Autodesk Fusion 360 part; units mm, degrees
sketch "Sketch1" plane through (0, 0, 0) normal (0, 0, 1) x (1, 0, 0)
  circle A0 centre (0, 0) radius 11
  dimension "d1" = 22
extrude "Extrude1" add sketch "Sketch1" along normal blind 2.5
sketch "Sketch2" plane through (0, 0, 2.5) normal (0, 0, 1) x (-1, 0, 0)
  circle A0 centre (0, 0) radius 11
  circle A1 centre (0, 0) radius 5.5
  dimension "d4" = 11
extrude "Extrude2" add sketch "Sketch2" along normal blind 8 contours A1
sketch "Sketch3" plane through (0, 0, 2.5) normal (0, 0, 1) x (-1, 0, 0)
  circle A0 centre (0, 0) radius 5.5
  circle A1 centre (0, 0) radius 11
  circle A2 centre (5.6569, -5.6569) radius 1.4
  circle A3 centre (5.6569, 5.6569) radius 1.4
  circle A4 centre (-5.6569, 5.6569) radius 1.4
  circle A5 centre (-5.6569, -5.6569) radius 1.4
  line L0 (0, 0) -> (7.7782, -7.7782) construction
  line L1 (0, 0) -> (11, 0) construction
  dimension "d7" = 2.8
  dimension "d8" = 8
  dimension "d10" = 360
  dimension "d27" = 45
extrude "Extrude3" cut sketch "Sketch3" against normal through all contours A2 | A3 | A4 | A5
sketch "Sketch4" plane through (0, 0, 10.5) normal (0, 0, 1) x (-1, 0, 0)
  circle A0 centre (0, 0) radius 5.5
  circle A1 centre (0, 0) radius 1.1
  dimension "d12" = 2.2
extrude "Extrude4" cut sketch "Sketch4" against normal through all contours A1
chamfer "Chamfer1" distance 3 angle 45 1 edges at (5.1278, 1.9889, 10.5)
Build history of the part. All positions in model axes, mm. A direction names the side the tool comes from. Give positions to 0.01 mm unless a question says otherwise; leave off trailing zeros. Order: outer loops, then holes, each group sorted by start corner. A loop starts at its lowest first (then second) coordinate and runs counter-clockwise, first axis right, second up. Notation, with made-up numbers: M 1.5,42.25 L 18.5,42.25 A21 cw 18.5,78.25 Z; hole C 40.5,-10 d3. An arc over 180 degrees is marked long. Return JSON: item names as keys, results as strings.
Q1. Band-saw the part on C-C (z = 9). Give the cut face in (x, y).
Answer list:
{"outline": "C 0,0 d8; hole C 0,0 d2.2"}
Q2. 3-axis set-ups, long thin cutter, end or side, ignore diameter. For faces 1 (the face through (-4.625, -6.603, 1.268)), 2 (the face through (-3, 5, 2.5)): which of +Z, -Z, +X, -X, +Y, -Y reach the whole face in a straight line?
Answer list:
{"face 1": "+Z, -Z", "face 2": "+Z"}
Q3. Flat gauge pins, fed straight in: pin 1 (3 mm diameter, centred on x = 5.66, y = 5.66, fed in from +Z); pin 2 (12 mm diameter, centred on x = -6, y = 8, fed in from +Z); pin 3 (3 mm diameter, centred on y = -8, z = 1, fed in from -X). Where does each tip first touch, or does it go through?
Answer list:
{"pin 1": "stops at z = 2.5", "pin 2": "stops at z = 9", "pin 3": "stops at x = -8.87"}
Q4. Band-saw the part on A-A (x = 0). Give the cut face in (y, z).
Answer list:
{"outline": "M -11,0 L -1.1,0 L -1.1,10.5 L -2.5,10.5 L -5.5,7.5 L -5.5,2.5 L -11,2.5 Z; M 1.1,0 L 11,0 L 11,2.5 L 5.5,2.5 L 5.5,7.5 L 2.5,10.5 L 1.1,10.5 Z"}
Q5. Two-plate mould, pull along Y, no slides. Class faces 3 (the face through (4.904, -6.837, 1.268)), 4 (the face through (1.19, -5.37, 4.96)), 5 (the face through (0, -2, 0)): pulls with the +Y half, pulls with the -Y half, needs draft (parallel to the pull), parting line crosses it, or undercut.
Answer list:
{"face 3": "undercut", "face 4": "parting line crosses it", "face 5": "needs draft"}
Q6. Wall check: probe 1 along Y at (x, z) = (0, 6); probe 2 along Z at (x, y) = (-5.25, -1.75); probe 3 along X at (y, z) = (5.25, 1.75). Give the ranges that are in metal, low to high. Write a range as from..to.
Answer list:
{"probe 1": "y = -5.5..-1.1, 1.1..5.5", "probe 2": "z = 0..2.5", "probe 3": "x = -9.67..-7, -4.32..4.32, 7..9.67"}
Q7. Band-saw the part on D-D (z = 5.75). Give the cut face in (x, y), then the cut area to 3 significant figures.
Answer list:
{"outline": "C 0,0 d11; hole C 0,0 d2.2", "area": "91.2 mm^2"}
